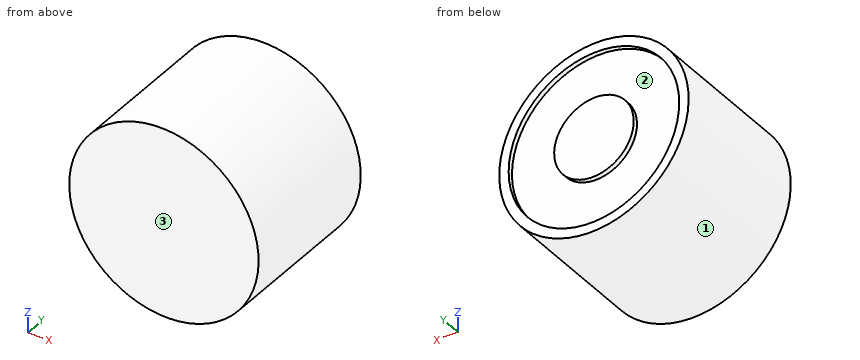
from build123d import *

# Parameters (mm, degrees)
SKETCH1_R           = 10
BOSS_EXTRUDE1_DEPTH = 15
SKETCH2_R           = 10
SKETCH2_R_2         = 9.008877903
BOSS_EXTRUDE2_DEPTH = 0.5
SKETCH3_R           = 4.201144216
BOSS_EXTRUDE3_DEPTH = 0.5


with BuildPart() as part:
    # Sketch1 → Boss-Extrude1 (new body)
    with BuildSketch(Plane(origin=(0, 0, 0), x_dir=(1, 0, 0), z_dir=(0, 1, 0))):
        with Locations(Location((0, 0, 0), (0, 0, 270))):
            Circle(SKETCH1_R)
    extrude(amount=BOSS_EXTRUDE1_DEPTH)

    # Sketch2 → Boss-Extrude2 (add)
    with BuildSketch(Plane(origin=(0, 15, 0), x_dir=(1, 0, 0), z_dir=(0, 1, 0))):
        with Locations(Location((0, 0, 0), (0, 0, 270))):
            Circle(SKETCH2_R)
        with Locations(Location((0, 0, 0), (0, 0, 270))):
            Circle(SKETCH2_R_2, mode=Mode.SUBTRACT)
    extrude(amount=BOSS_EXTRUDE2_DEPTH)

    # Sketch3 → Boss-Extrude3 (add)
    with BuildSketch(Plane(origin=(0, 15, 0), x_dir=(1, 0, 0), z_dir=(0, 1, 0))):
        with Locations(Location((0, 0, 0), (0, 0, 270))):
            Circle(SKETCH3_R)
    extrude(amount=BOSS_EXTRUDE3_DEPTH)


solid = part.part
Could you check a few things on this model? Use its own coordinates, in mm. Face numbers are marked on the shaded views. Round coordinates to 2 decimals unless told otherwise and drop trailing zeros. Write each loop counter-clockwise with the first axis right and the second up, starting at its lowest first coordinate (ties: lowest second). Pieces come first, ordered by that corner, then holes. Notation, with made-up numbers: (40, -35.75) -> (51, -35.75) arc R16 cw to (51, -29.75) -> close; hole circle Ø4 at (84.25, 25). An arc over 180 degrees is marked (long way). Use a Markdown table: item, result.
1. If we section it at A-A (x = 0): List the corners of the cut face in (y, z) for me.
Answer key:
| item | result |
|---|---|
| outline | (0, -10) -> (15.5, -10) -> (15.5, -9.01) -> (15, -9.01) -> (15, -4.2) -> (15.5, -4.2) -> (15.5, 4.2) -> (15, 4.2) -> (15, 9.01) -> (15.5, 9.01) -> (15.5, 10) -> (0, 10) -> close |
2. If we section it at C-C (y = 3.25): List the corners of the cut face in (x, z) for me.
Answer key:
| item | result |
|---|---|
| outline | circle Ø20 at (0, 0) |
3. For pin 1 Ø2 at (y, z) = (3.5, -4.5) entering from -X; pin 2 Ø1.5 at (x, z) = (0.5, -1) entering from -Y; pin 3 Ø1 at (x, y) = (4, 13) entering from +Z; pin 4 Ø2 at (x, y) = (2.5, 12.5) entering from -Z, each with a flat end and sliding along its axis, tell me the tip position at first contact or that it passes through.
Answer key:
| item | result |
|---|---|
| pin 1 | stops at x = -9.37 |
| pin 2 | stops at y = 0 |
| pin 3 | stops at z = 9.37 |
| pin 4 | stops at z = -9.89 |
4. If we section it at D-D (z = 8.5): List the corners of the cut face in (x, y) for me, then the cut area to 3 significant figures.
Answer key:
| item | result |
|---|---|
| outline | (-5.27, 0) -> (5.27, 0) -> (5.27, 15.5) -> (2.98, 15.5) -> (2.98, 15) -> (-2.98, 15) -> (-2.98, 15.5) -> (-5.27, 15.5) -> close |
| area | 160 mm^2 |
5. If we section it at B-B (z = 0): List the corners of the cut face in (x, y) for me, then the cut area to 3 significant figures.
Answer key:
| item | result |
|---|---|
| outline | (-10, 0) -> (10, 0) -> (10, 15.5) -> (9.01, 15.5) -> (9.01, 15) -> (4.2, 15) -> (4.2, 15.5) -> (-4.2, 15.5) -> (-4.2, 15) -> (-9.01, 15) -> (-9.01, 15.5) -> (-10, 15.5) -> close |
| area | 305 mm^2 |
6. Please list where these lines run through material, in increasing order: probe 1 along X at (y, z) = (15.3, 0); probe 2 along Y at (x, z) = (-5.75, 5); probe 3 along Z at (x, y) = (-2.75, 8.25).
Answer key:
| item | result |
|---|---|
| probe 1 | x = -10 to -9.01, -4.2 to 4.2, 9.01 to 10 |
| probe 2 | y = 0 to 15 |
| probe 3 | z = -9.61 to 9.61 |
7. We'd pull the mould along X, two halves only. Please class the marked faces 1, 2 and 3: +X half, -X half, draft (parallel to the pull), parting line (faces both ways), or undercut.
Answer key:
| item | result |
|---|---|
| face 1 | parting line |
| face 2 | undercut |
| face 3 | draft |
